Can you work these out from the model? Positions are in its coordinate system, mm. Face numbers are marked on the shaded views. A direction names the side the tool comes from. Coordinates: 2 decimals unless noted, no trailing zeros. Order: outer loops, then holes, each group sorted by start corner. A loop starts at its lowest first (then second) coordinate and runs counter-clockwise, first axis right, second up. Notation, with made-up numbers: (62, 75.25) -> (69, 75.25) arc R6 cw to (69, 83.25) -> close; hole circle Ø4 at (18, -18.5). An arc over 180 degrees is marked (long way). Write item = value, one per line.
Autodesk Inventor part; units mm, degrees
ref_plane "YZ Plane" through (0, 0, 0) normal (1, 0, 0) x (0, 1, 0)
ref_plane "XZ Plane" through (0, 0, 0) normal (0, 1, 0) x (-1, 0, 0)
ref_plane "XY Plane" through (0, 0, 0) normal (0, 0, 1) x (1, 0, 0)
sketch "Sketch1" plane through (0, 0, 0) normal (0, 0, 1) x (1, 0, 0)
  line L0 (-15, 15) -> (15, 15)
  line L1 (15, 15) -> (15, -15)
  line L2 (15, -15) -> (-15, -15)
  line L3 (-15, -15) -> (-15, 15)
  point P0 (0, 0)
  point P1 (0, 15)
  point P2 (-15, 0)
  dimension "d0" = 30
  dimension "d1" = 30
extrude "Extrusion1" add sketch "Sketch1" along normal blind 30
sketch "Sketch4" plane through (0, 0, 0) normal (0, 0, -1) x (-1, 0, 0)
  line L0 (5, -15) -> (-5, -15)
  line L1 (-5, -15) -> (-5, 15)
  line L2 (-5, 15) -> (5, 15)
  line L3 (5, 15) -> (5, -15)
  line L4 (15, -15) -> (-15, -15)
  line L5 (-15, 15) -> (15, 15)
  point P0 (0, 0)
  point P1 (0, -15)
  dimension "d8" = 10
extrude "Extrusion3" cut sketch "Sketch4" against normal blind 15
sketch "Sketch5" plane through (15, -15, 0) normal (1, 0, 0) x (0, 0, -1)
  line L0 (0, 0) -> (0, 30)
  point P0 (0, 15)
  point P1 (-5, 15)
  point P2 (0, 15)
  dimension "d11" = 5
hole "Hole1" at (15, 0, 5) direction (-1, 0, 0) diameter 5.5 end through all
sketch "Sketch8" plane through (15, 15, 30) normal (0, 1, 0) x (1, 0, 0)
  line L0 (0, 0) -> (-30, 0)
  line L1 (0, 30) -> (0, 0)
  line L2 (0, 30) -> (-10, 30)
  line L3 (-10, 30) -> (-10, 15)
  line L4 (-10, 15) -> (-20, 15)
  line L5 (-20, 15) -> (-20, 30)
  line L6 (-20, 30) -> (-30, 30)
  circle A0 centre (-25, 5) radius 2.25
  circle A1 centre (-5, 5) radius 2.25
  line L7 (-30, 30) -> (-30, 0)
  point P0 (-15, 30)
  dimension "d28" = 4.5
  dimension "d30" = 5
  dimension "d31" = 5
  dimension "d32" = 5
extrude "Extrusion6" cut sketch "Sketch8" against normal through all contours A0 | A1
properties part number "0005-10-019 intinzator y"
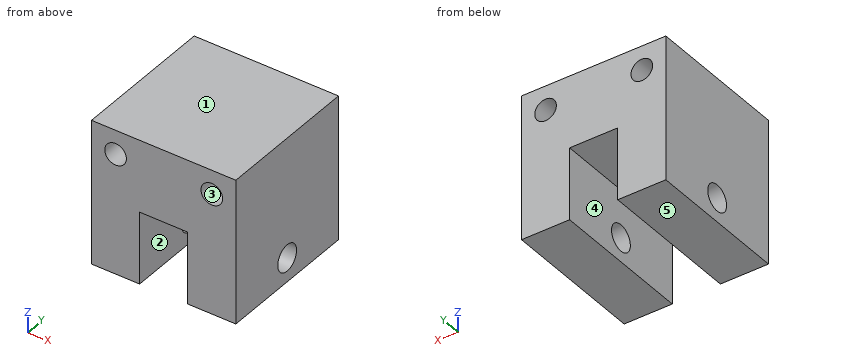
Item 1: If we mould it in two halves opening along Z, with no side actions, what happens to the marked faces 1, 2 and 3? For each: pulls with the +Z half, pulls with the -Z half, needs draft (parallel to the pull), parting line crosses it, or undercut.
A:
face_1 = pulls with the +Z half
face_2 = needs draft
face_3 = undercut
Item 2: If I drill on probe 1 along X at (y, z) = (7.5, 25); probe 2 along Y at (x, z) = (12.75, 5); probe 3 along Z at (x, y) = (10, 12.75), over which ranges is the centre line in solid material (lowest first)?
A:
probe_1 = -15 to -12.25, -7.75 to 7.75, 12.25 to 15
probe_2 = -15 to -2.75, 2.75 to 15
probe_3 = 0 to 22.75, 27.25 to 30
Item 3: I want a section at D-D, the plane z = 5. Please give me the cut outline in (x, y), plus the area to 3 significant figures.
A:
outline = (-15, -15) -> (-5, -15) -> (-5, -2.75) -> (-15, -2.75) -> close; (-15, 2.75) -> (-5, 2.75) -> (-5, 15) -> (-15, 15) -> close; (5, -15) -> (15, -15) -> (15, -2.75) -> (5, -2.75) -> close; (5, 2.75) -> (15, 2.75) -> (15, 15) -> (5, 15) -> close
area = 490 mm2
Item 4: For the marked faces 4 and 5, which set-ups out of +Z, -Z, +X, -X, +Y, -Y let a thin tool reach every point of the face, with its end or its side?
A:
face_4 = -Z, +Y, -Y
face_5 = -Z, +X, -X, +Y, -Y
Item 5: I want a section at A-A, the plane z = 8.5. Please give me the cut outline in (x, y), plus the area to 3 significant figures.
A:
outline = (-15, -15) -> (-5, -15) -> (-5, 15) -> (-15, 15) -> close; (5, -15) -> (15, -15) -> (15, 15) -> (5, 15) -> close
area = 600 mm2
Item 6: I want a section at B-B, the plane x = -10. Please give me the cut outline in (y, z).
A:
outline = (-15, 0) -> (15, 0) -> (15, 22.75) -> (-15, 22.75) -> close; (-15, 27.25) -> (15, 27.25) -> (15, 30) -> (-15, 30) -> close; hole circle Ø5.5 at (0, 5)
Item 7: I want a section at C-C, the plane y = -9. Please give me the cut outline in (x, z), plus the area to 3 significant figures.
A:
outline = (-15, 0) -> (-5, 0) -> (-5, 15) -> (5, 15) -> (5, 0) -> (15, 0) -> (15, 30) -> (-15, 30) -> close; hole circle Ø4.5 at (-10, 25); hole circle Ø4.5 at (10, 25)
area = 718 mm2
Item 8: I'm going to push flat-ended pins straight in: P1, Ø12, axis at x = -7, y = 10.5, coming from the -Z side; P2, Ø1, axis at x = 4, y = 12, coming from the -Z side. Where does each tip first touch, or does it pass through?
A:
P1 = 0
P2 = 15
